```python
from build123d import *

# Parameters (mm, degrees)
F0_W     = 177.8
F0_H     = 152.4
F1_DEPTH = 50.8
F2_R     = 63.5
F3_DEPTH = 50.8
F4_R     = 5.08
F5_T     = -2.54


with BuildPart() as f1:
    # F0 (on Front) → F1 (new body)
    with BuildSketch(Plane.XZ):
        Rectangle(F0_W, F0_H)
    extrude(amount=F1_DEPTH)

    # F2 (on face) → F3 (join)
    with BuildSketch(Plane.XZ.offset(50.8)):
        Circle(F2_R)
    extrude(amount=F3_DEPTH)

    # F4
    f4_edges = [f1.edges().sort_by_distance(p)[0] for p in [
        (-63.5, -101.6, 0),
        (-63.5, -50.8, 0),
        (88.9, -50.8, 0),
        (0, -50.8, -76.2),
        (0, -50.8, 76.2),
        (-88.9, -50.8, 0),
        (88.9, -25.4, 76.2),
        (-88.9, -25.4, 76.2),
        (-88.9, -25.4, -76.2),
        (88.9, -25.4, -76.2),
    ]]
    fillet(f4_edges, radius=F4_R)

    # F5
    f5_openings = [f1.faces().sort_by_distance(p)[0] for p in [
        (0, 0, 0),
    ]]
    offset(amount=F5_T, openings=f5_openings)


solid = f1.part
```
Check sheet for the modelled part. Datum: model origin and axes. Units: mm. A direction names the side the tool comes from. Round coordinates to 2 decimals unless told otherwise and drop trailing zeros. Write each loop counter-clockwise with the first axis right and the second up, starting at its lowest first coordinate (ties: lowest second). Pieces come first, ordered by that corner, then holes. Notation, with made-up numbers: (41, 79) -> (56, 79) arc R24 cw to (56, 89) -> close; hole circle Ø3 at (-9.5, 86.5). An arc over 180 degrees is marked (long way). One line per question, with ' | ' between items. Start each with the question number.
1. Release check for a two-part mould opening along Z. For faces 1 (the face through (-1, -23, 73.66)), 2 (the face through (-1, -23, -73.66)), 3 (the face through (-1, -23, -76.2)), 4 (the face through (-88.9, -23, -1)) record: +Z half, -Z half, draft (parallel to the pull), parting line (faces both ways), or undercut.
2. Sectioned sample at D-D, the plane x = 0. Record the cut outline in (y, z), then the cut area to 3 significant figures.
3. Sectioned sample at C-C, the plane x = 77. Record the cut outline in (y, z), then the cut area to 3 significant figures.
4. Sectioned sample at B-B, the plane z = 0. Record the cut outline in (x, y), then the cut area to 3 significant figures.
5. Depth check by flat-ended pin: pin 1 (8 mm diameter, centred on x = -1.5, y = -66, fed in from -Z); pin 2 (2 mm diameter, centred on x = -17.5, y = -53.5, fed in from -Z); pin 3 (3 mm diameter, centred on x = 8.5, z = 29, fed in from +Y); pin 4 (2 mm diameter, centred on x = 65, y = -54, fed in from -Z) (3 decimals). Enter the tip coordinate at first touch or a pass-through.
6. Scan lines: line 1 along Z through (x, y) = (-71, -14); line 2 along Z through (x, y) = (2, -63); line 3 along X through (y, z) = (-14, -42.5). Record each from-to range of solid material in increasing order. Write a range as from..to.
7. Set-up check for faces 5 (the face through (-57, -48.26, 48)), 6 (the face through (-57, -50.8, 48)), 7 (the face through (88.9, -23, -1)): record each of +Z, -Z, +X, -X, +Y, -Y from which the full face is reachable in a straight line by a thin tool's end or side.
8. Sectioned sample at A-A, the plane y = -29. Record the cut outline in (x, z), then the cut area to 4 significant figures.
Taken from the geometry:
1) face 1: undercut | face 2: undercut | face 3: -Z half | face 4: draft
2) outline: (-101.6, -58.42) arc R5.08 ccw to (-96.52, -63.5) -> (-55.88, -63.5) arc R5.08 cw to (-50.8, -68.58) -> (-50.8, -71.12) arc R5.08 ccw to (-45.72, -76.2) -> (0, -76.2) -> (0, -73.66) -> (-45.72, -73.66) arc R2.54 cw to (-48.26, -71.12) -> (-48.26, -68.58) arc R7.62 ccw to (-55.88, -60.96) -> (-96.52, -60.96) arc R2.54 cw to (-99.06, -58.42) -> (-99.06, 58.42) arc R2.54 cw to (-96.52, 60.96) -> (-55.88, 60.96) arc R7.62 ccw to (-48.26, 68.58) -> (-48.26, 71.12) arc R2.54 cw to (-45.72, 73.66) -> (0, 73.66) -> (0, 76.2) -> (-45.72, 76.2) arc R5.08 ccw to (-50.8, 71.12) -> (-50.8, 68.58) arc R5.08 cw to (-55.88, 63.5) -> (-96.52, 63.5) arc R5.08 ccw to (-101.6, 58.42) -> close | area: 860 mm^2
3) outline: (-50.8, -71.12) arc R5.08 ccw to (-45.72, -76.2) -> (0, -76.2) -> (0, -73.66) -> (-45.72, -73.66) arc R2.54 cw to (-48.26, -71.12) -> (-48.26, 71.12) arc R2.54 cw to (-45.72, 73.66) -> (0, 73.66) -> (0, 76.2) -> (-45.72, 76.2) arc R5.08 ccw to (-50.8, 71.12) -> close | area: 624 mm^2
4) outline: (-88.9, -45.72) arc R5.08 ccw to (-83.82, -50.8) -> (-68.58, -50.8) arc R5.08 cw to (-63.5, -55.88) -> (-63.5, -96.52) arc R5.08 ccw to (-58.42, -101.6) -> (58.42, -101.6) arc R5.08 ccw to (63.5, -96.52) -> (63.5, -55.88) arc R5.08 cw to (68.58, -50.8) -> (83.82, -50.8) arc R5.08 ccw to (88.9, -45.72) -> (88.9, 0) -> (86.36, 0) -> (86.36, -45.72) arc R2.54 cw to (83.82, -48.26) -> (68.58, -48.26) arc R7.62 ccw to (60.96, -55.88) -> (60.96, -96.52) arc R2.54 cw to (58.42, -99.06) -> (-58.42, -99.06) arc R2.54 cw to (-60.96, -96.52) -> (-60.96, -55.88) arc R7.62 ccw to (-68.58, -48.26) -> (-83.82, -48.26) arc R2.54 cw to (-86.36, -45.72) -> (-86.36, 0) -> (-88.9, 0) -> close | area: 924 mm^2
5) pin 1: stops at z = -63.5 | pin 2: stops at z = -62.42 | pin 3: stops at y = -99.06 | pin 4: passes through
6) line 1: z = -76.2..-73.66, 73.66..76.2 | line 2: z = -63.47..-60.93, 60.93..63.47 | line 3: x = -88.9..-86.36, 86.36..88.9
7) face 5: +Y | face 6: -Y | face 7: +Z, -Z, +X, +Y, -Y
8) outline: (-88.9, -71.12) arc R5.08 ccw to (-83.82, -76.2) -> (83.82, -76.2) arc R5.08 ccw to (88.9, -71.12) -> (88.9, 71.12) arc R5.08 ccw to (83.82, 76.2) -> (-83.82, 76.2) arc R5.08 ccw to (-88.9, 71.12) -> close; hole (-86.36, -71.12) arc R2.54 ccw to (-83.82, -73.66) -> (83.82, -73.66) arc R2.54 ccw to (86.36, -71.12) -> (86.36, 71.12) arc R2.54 ccw to (83.82, 73.66) -> (-83.82, 73.66) arc R2.54 ccw to (-86.36, 71.12) -> close | area: 1,635 mm^2
